For this review, take the finished solid that the model builds, in its own axes (mm). Face numbers are marked on the shaded views. A direction names the side the tool comes from. Round coordinates to 2 decimals unless told otherwise and drop trailing zeros. Write each loop counter-clockwise with the first axis right and the second up, starting at its lowest first coordinate (ties: lowest second). Pieces come first, ordered by that corner, then holes. Notation, with made-up numbers: (-14, 11) - (26, 11) arc R24 cw to (26, 42) - close; hole circle Ø11 at (2, 22). An arc over 180 degrees is marked (long way). One line per item, written item: value. Start each with the question number.
Q1. Add section B-B on y = -9.5. Write out the cut boundary in (x, z).
Q2. For probe 1 along Z at (x, y) = (0, -33); probe 2 along Z at (x, y) = (0, -24.5); probe 3 along Y at (x, z) = (-7.5, -9), list the stretches that pass through material, from the lowest coordinate up.
Q3. Clearance check with flat-ended pins moving along their axes: pin 1 Ø1.5 at (y, z) = (-34, 6.5) entering from +X; pin 2 Ø8 at (x, z) = (0, 0) entering from +Y; pin 3 Ø10 at (y, z) = (-47, -1) entering from +X. State where each tip first meets the part, or that it passes through.
Q4. Add section D-D on x = 13. Write out the cut boundary in (y, z), and give its area (3 significant figures).
Q5. Tool access review of the marked faces 4 and 5: name each direction out of +Z, -Z, +X, -X, +Y, -Y from which nothing blocks a thin tool from reaching the whole face with its end or side.
Q6. Mouldability with a two-part tool opening along X and no side actions: class the marked faces 1, 2 and 3 as +X half, -X half, draft (parallel to the pull), parting line (faces both ways), or undercut.
```python
from build123d import *

# Parameters (mm, degrees)
F0_W     = 30
F0_H     = 30
F1_DEPTH = 30
F2_R     = 10
F3_DEPTH = 30
F4_R     = 5
F5_DEPTH = 60.001
F6_R     = 4.99999


# Not quite as in the source:
# - a fillet or chamfer is up to 0.001 mm smaller than in the source, because OpenCascade refuses the exact size


with BuildPart() as f1:
    # F0 (on Front) → F1 (new body)
    with BuildSketch(Plane.XZ):
        Rectangle(F0_W, F0_H)
    extrude(amount=F1_DEPTH)

    # F2 (on face) → F3 (join)
    with BuildSketch(Plane.XZ.offset(30)):
        Circle(F2_R)
    extrude(amount=F3_DEPTH)

    # F4 (on face) → F5 (cut, through all)
    with BuildSketch(Plane.XZ.offset(60)):
        Circle(F4_R)
    extrude(amount=-F5_DEPTH, mode=Mode.SUBTRACT)

    # F6 (radius 5 in the source; OpenCascade refuses exactly that, so slightly less here)
    f6_edges = [f1.edges().sort_by_distance(p)[0] for p in [
        (0, -30, 15),
        (-15, -30, 0),
        (0, -30, -15),
        (15, -30, 0),
        (15, -15, 15),
        (15, -15, -15),
        (0, 0, -15),
        (-15, 0, 0),
        (15, 0, 0),
        (0, 0, 15),
        (-15, -15, 15),
        (-10, -60, 0),
        (-15, -15, -15),
    ]]
    fillet(f6_edges, radius=F6_R)


solid = f1.part
```
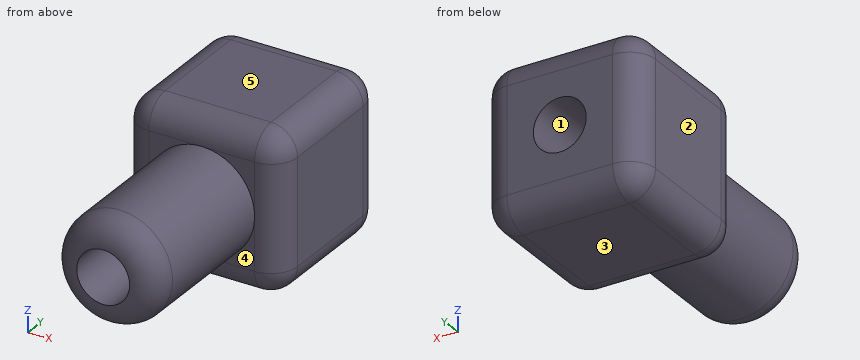
Result set:
1. outline: (-15, -10) arc R5 ccw to (-10, -15) - (10, -15) arc R5 ccw to (15, -10) - (15, 10) arc R5 ccw to (10, 15) - (-10, 15) arc R5 ccw to (-15, 10) - close; hole circle Ø10 at (0, 0)
2. probe 1: z = -10 to -5, 5 to 10
2. probe 2: z = -15 to -5, 5 to 15
2. probe 3: y = -30 to 0
3. pin 1: stops at x = 8.18
3. pin 2: passes through
3. pin 3: stops at x = 10
4. outline: (-29, -10) arc R4 ccw to (-25, -14) - (-5, -14) arc R4 ccw to (-1, -10) - (-1, 10) arc R4 ccw to (-5, 14) - (-25, 14) arc R4 ccw to (-29, 10) - close
4. area: 770 mm^2
5. face 4: -Y
5. face 5: +Z, +X, -X, +Y, -Y
6. face 1: undercut
6. face 2: -X half
6. face 3: draft
